Read the model definition and answer for the solid it produces. Units are mm, in the model's axes. Face numbers are marked on the shaded views. A direction names the side the tool comes from. Coordinates: 2 decimals unless noted, no trailing zeros. Write each loop counter-clockwise with the first axis right and the second up, starting at its lowest first coordinate (ties: lowest second). Pieces come first, ordered by that corner, then holes. Notation, with made-up numbers: (19.25, 83) - (37.25, 83) arc R20 ccw to (37.25, 89) - close; hole circle Ø6 at (70.5, 12.5). An arc over 180 degrees is marked (long way). Return JSON: item names as keys, results as strings.
```python
from build123d import *

# Parameters (mm, degrees)
BOSS_EXTRUDE1_DEPTH             = 5
TAP_DRILL_FOR_M2X0_4_TAP1_D     = 1.6
TAP_DRILL_FOR_M2X0_4_TAP1_DEPTH = 5


with BuildPart() as part:
    # Sketch1 → Boss-Extrude1 (new body)
    with BuildSketch(Plane(origin=(0, 0, 0), x_dir=(0, 0, -1), z_dir=(1, 0, 0))):
        Polygon((0, 4), (0, 8.3), (36.4, 8.3), (36.4, 4), (28.4, 4), (28.4, 0), (4, 0), (4, 4), align=None)
    extrude(amount=BOSS_EXTRUDE1_DEPTH)

    # Tap Drill for M2x0.4 Tap1
    with Locations(Plane(origin=(0, 0, 0), x_dir=(-1, 0, 0), z_dir=(0, -1, 0))):
        with Locations((-2.5, 9), (-2.5, 23.4)):
            Hole(TAP_DRILL_FOR_M2X0_4_TAP1_D / 2, depth=TAP_DRILL_FOR_M2X0_4_TAP1_DEPTH)


solid = part.part
```
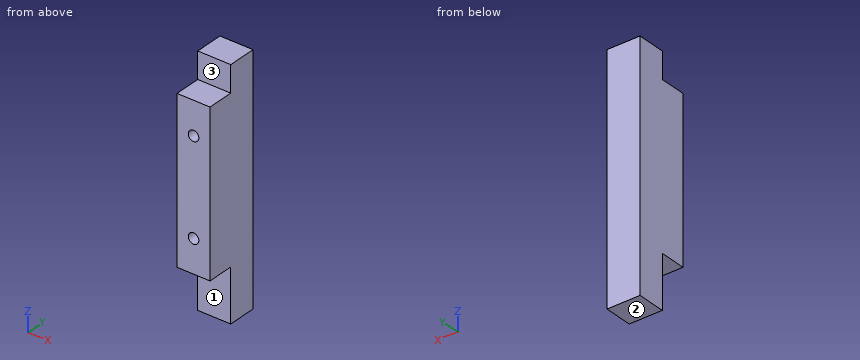
(1) Straight lines are drawn through the part: line 1 (Z direction, x = 2.5, y = 2.9); line 2 (X direction, y = 3.7, z = -23.4); line 3 (Z direction, x = 2.1, y = 0.5). For each, find the intervals that lie inside material, in ascending order. Write a range as from..to.
Answer:
{"line 1": "-28.4..-24.2, -22.6..-9.8, -8.2..-4", "line 2": "0..1.7, 3.3..5", "line 3": "-28.4..-24.09, -22.71..-9.69, -8.31..-4"}
(2) A cutting plane is placed at C-C (z = -9). Determine the outline of the cut face in (x, y), and give its area (3 significant figures).
Answer:
{"outline": "(0, 0) - (1.7, 0) - (1.7, 5) - (3.3, 5) - (3.3, 0) - (5, 0) - (5, 8.3) - (0, 8.3) - close", "area": "33.5 mm²"}
(3) A cutting plane is placed at B-B (x = 2.5). Determine the outline of the cut face in (y, z).
Answer:
{"outline": "(0, -28.4) - (4, -28.4) - (4, -36.4) - (8.3, -36.4) - (8.3, 0) - (4, 0) - (4, -4) - (0, -4) - (0, -8.2) - (5, -8.2) - (5, -9.8) - (0, -9.8) - (0, -22.6) - (5, -22.6) - (5, -24.2) - (0, -24.2) - close"}
(4) A cutting plane is placed at A-A (y = 1.5). Determine the outline of the cut face in (x, z), and give its area (3 significant figures).
Answer:
{"outline": "(0, -28.4) - (5, -28.4) - (5, -4) - (0, -4) - close; hole circle Ø1.6 at (2.5, -23.4); hole circle Ø1.6 at (2.5, -9)", "area": "118 mm²"}
(5) Which of the six approach directions +Z, -Z, +X, -X, +Y, -Y give full straight-line access (tool end or side, diameter ignored) to the marked faces 1, 2 and 3?
Answer:
{"face 1": "-Z, +X, -X, -Y", "face 2": "-Z, +X, -X, +Y, -Y", "face 3": "+Z, +X, -X, -Y"}
(6) Flat-ended cylindrical pins translate along their axes: P1, Ø0.8, axis at x = 2.5, z = -9, coming from the -Y side; P2, Ø2.5, axis at x = 2.5, z = -33.5, coming from the -Y side; P3, Ø3, axis at x = 3, y = 1.5, coming from the -Z side. Find the tip coordinate at first contact, or state that the pin passes through.
Answer:
{"P1": "y = 5", "P2": "y = 4", "P3": "z = -28.4"}
